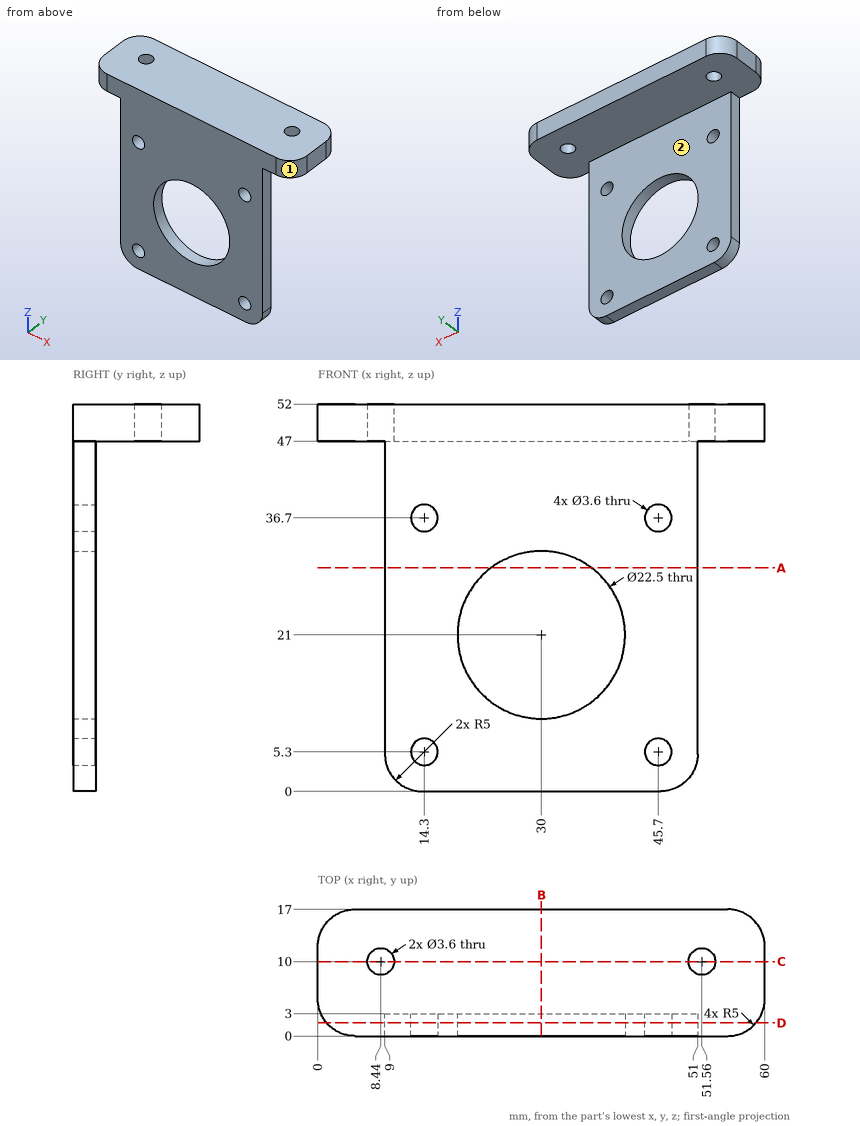
Can you work these out from the drawing? Everything is in mm from the part's minimum corner. A direction names the side the tool comes from. Coordinates: 2 decimals unless noted, no trailing zeros. Order: outer loops, then holes, each group sorted by start corner. A loop starts at its lowest first (then second) coordinate and runs counter-clockwise, first axis right, second up. Notation, with made-up numbers: M -17.75,9.5 L 29.25,9.5 A18 cw 29.25,34.5 Z; hole C 30,-4.5 d8. An arc over 180 degrees is marked long. Answer as CSV lines item,"result". Start each with the question number.
1. On a 3-axis mill with a long thin cutter (end or side, diameter ignored), from which of +Z, -Z, +X, -X, +Y, -Y can I reach the whole of each face in a straight line? I mean the marked faces 1 and 2. Say none if no direction works.
2. I want a section at A-A, the plane z = 30. Write out the boundary of the cut face in (x, y).
3. I want a section at D-D, the plane y = 1.75. Write out the boundary of the cut face in (x, z), and give its area (3 significant figures).
4. I need wall thicknesses on line 1 (X direction, y = 10, z = 50.1); line 2 (X direction, y = 9, z = 49.5) (1 decimal); line 3 (Z direction, x = 10, y = 6). Which ranges of each line are inside material? Lowest first, please. Write a range as [from, to].
5. I want a section at B-B, the plane x = 30. Write out the boundary of the cut face in (y, z).
6. I want a section at C-C, the plane y = 10. Write out the boundary of the cut face in (x, z).
7. For pin 1 (8 mm diameter, centred on x = 28.5, z = 40, fed in from +Y); pin 2 (3 mm diameter, centred on x = 51.56, y = 10, fed in from +Z); pin 3 (4.5 mm diameter, centred on x = 45.7, z = 5.3, fed in from -Y); pin 4 (1.5 mm diameter, centred on y = 1.5, z = 25, fed in from +X), each with a flat end and sliding along its axis, tell me the tip position at first contact or that it passes through.
Recorded:
1,face 1,"+Z, -Z, +X, -Y"
1,face 2,"-Z, +X, -X, +Y"
2,outline,"M 9,0 L 23.25,0 L 23.25,3 L 9,3 Z; M 36.75,0 L 51,0 L 51,3 L 36.75,3 Z"
3,outline,"M 1.2,47 L 9,47 L 9,5 A5 ccw 14,0 L 46,0 A5 ccw 51,5 L 51,47 L 58.8,47 L 58.8,52 L 1.2,52 Z; hole C 14.3,5.3 d3.6; hole C 14.3,36.7 d3.6; hole C 30,21 d22.5; hole C 45.7,5.3 d3.6; hole C 45.7,36.7 d3.6"
3,area,"1,810 mm2"
4,line 1,"x = [0, 6.64], [10.24, 49.76], [53.36, 60]"
4,line 2,"x = [0, 6.9], [9.9, 50.1], [53.1, 60]"
4,line 3,"z = [47, 52]"
5,outline,"M 0,0 L 3,0 L 3,9.75 L 0,9.75 Z; M 0,32.25 L 3,32.25 L 3,47 L 17,47 L 17,52 L 0,52 Z"
6,outline,"M 0,47 L 6.64,47 L 6.64,52 L 0,52 Z; M 10.24,47 L 49.76,47 L 49.76,52 L 10.24,52 Z; M 53.36,47 L 60,47 L 60,52 L 53.36,52 Z"
7,pin 1,"stops at y = 3"
7,pin 2,"passes through"
7,pin 3,"stops at y = 0"
7,pin 4,"stops at x = 51"
